```python
from build123d import *

# Parameters (mm, degrees)
F0_W          = 114.3
F0_H          = 21.9340088606
F1_DEPTH      = 76.2
F1_DEPTH_BACK = 76.2
F2_T          = -2.54
F3_R          = 5.08
F4_R          = 6.35
F5_DEPTH      = 12.7
F6_R          = 6.35
F7_DEPTH      = 12.7


with BuildPart() as f1:
    # F0 (on Front) → F1 (new body, two sides)
    with BuildSketch(Plane.XZ) as f1_sk:
        Polygon((-57.15, -101.6), (-76.2, -101.6), (-57.15, -123.5340088606), align=None)
        Polygon((76.2, -101.6), (57.15, -101.6), (57.15, -123.5340088606), align=None)
        Polygon((-76.2, 101.6), (-76.2, -101.6), (-57.15, -101.6), (-57.15, -79.6659911394), (57.15, -79.6659911394), (57.15, -101.6), (76.2, -101.6), (76.2, 101.6), align=None)
        with Locations((0, -90.6329955697)):
            Rectangle(F0_W, F0_H)
        with Locations((0, -112.5670044303)):
            Rectangle(F0_W, F0_H)
    extrude(amount=-F1_DEPTH)
    extrude(f1_sk.sketch, amount=F1_DEPTH_BACK)

    # F2
    f2_openings = [f1.faces().sort_by_distance(p)[0] for p in [
        (0, 0, 101.6),
    ]]
    offset(amount=F2_T, openings=f2_openings)

    # F3
    f3_edges = [f1.edges().sort_by_distance(p)[0] for p in [
        (-66.675, 76.2, -112.567004),
        (-57.15, 0, -123.534009),
        (-66.675, -76.2, -112.567004),
        (-76.2, 0, -101.6),
        (57.15, 0, -123.534009),
        (66.675, 76.2, -112.567004),
        (76.2, 0, -101.6),
        (66.675, -76.2, -112.567004),
    ]]
    fillet(f3_edges, radius=F3_R)

    # F4 (on face) → F5 (join)
    with BuildSketch(Plane(origin=(-76.2, 0, 0), x_dir=(0, -1, 0), z_dir=(-1, 0, 0))):
        with Locations((-44.45, 69.85)):
            Circle(F4_R)
        with Locations((44.45, 69.85)):
            Circle(F4_R)
    extrude(amount=F5_DEPTH)

    # F6 (on face) → F7 (join)
    with BuildSketch(Plane.YZ.offset(76.2)):
        with Locations((-44.45, 69.85)):
            Circle(F6_R)
        with Locations((44.45, 69.85)):
            Circle(F6_R)
    extrude(amount=F7_DEPTH)


solid = f1.part
```
CAD build for the part. Positions are in the model's coordinates, mm. A direction names the side the tool comes from. Coordinates: 2 decimals unless noted, no trailing zeros. Loops run counter-clockwise (first coordinate to the right, second up) from the corner with the lowest first, then second, coordinate; pieces in that order, holes last. Notation, with made-up numbers: (22, 87) - (45, 87) arc R23 ccw to (45, 97) - close; hole circle Ø5 at (80.25, -15.5). An arc over 180 degrees is marked (long way). Use CSV: the item, a comma, the result in double quotes. Start each with the question number.
Q1. 3-axis set-ups, long thin cutter, end or side, ignore diameter. For faces 1 (the cylindrical face through (82.461, -41.036, 75.204)), 2 (the cylindrical face through (-82.461, -47.864, 75.204)), 3 (the cylindrical face through (66.17, 74.75, -110.82)), 4 (the flat face through (74, 34, 101.6)), 5 (the flat face through (-1, 1, -120.994)): which of +Z, -Z, +X, -X, +Y, -Y reach the whole face in a straight line?
Q2. Cut at B-B, the plane y = 32. List the corners of the cut face in (x, z).
Q3. Cut at A-A, the plane z = 58. List the corners of the cut face in (x, y), then the cut area to 3 significant figures.
Q4. Cut at C-C, the plane x = 25. List the corners of the cut face in (y, z).
Q5. Probe probe 1 along X at (y, z) = (4, 25); probe 2 along Z at (x, y) = (3.5, 54). List the from-to ranges inside material, lowest first. Write a range as from..to.
Q6. Two-plate mould, pull along Y, no slides. Class faces 6 (the flat face through (88.9, 44, 70)), 7 (the cylindrical face through (-65.872, 74.672, -111.282)), 8 (the flat face through (-1, -73.66, -8)): +Y half, -Y half, draft (parallel to the pull), parting line (faces both ways), or undercut.
Q7. Drop flat-ended pins along their axis: P1, Ø6, axis at y = 10, z = -13, coming from the -X side; P2, Ø1.5, axis at x = 57, y = 10.5, coming from the +Z side; P3, Ø1.5, axis at y = -21, z = 69.5, coming from the +X side. Give the stop position or say it passes through.
Here are the results:
1,face 1,"+X"
1,face 2,"-X"
1,face 3,"-Z, +X, +Y"
1,face 4,"+Z, +X, -X, +Y, -Y"
1,face 5,"+Z"
2,outline,"(-76.2, -99.7) arc R5.08 ccw to (-74.96, -103.03) - (-58.67, -121.79) arc R5.08 ccw to (-54.83, -123.53) - (54.83, -123.53) arc R5.08 ccw to (58.67, -121.79) - (74.96, -103.03) arc R5.08 ccw to (76.2, -99.7) - (76.2, 101.6) - (73.66, 101.6) - (73.66, -100.65) - (55.99, -120.99) - (-55.99, -120.99) - (-73.66, -100.65) - (-73.66, 101.6) - (-76.2, 101.6) - close"
3,outline,"(-76.2, -76.2) - (76.2, -76.2) - (76.2, 76.2) - (-76.2, 76.2) - close; hole (-73.66, -73.66) - (73.66, -73.66) - (73.66, 73.66) - (-73.66, 73.66) - close"
3,area,"1,520 mm2"
4,outline,"(-76.2, -123.53) - (76.2, -123.53) - (76.2, 101.6) - (73.66, 101.6) - (73.66, -120.99) - (-73.66, -120.99) - (-73.66, 101.6) - (-76.2, 101.6) - close"
5,probe 1,"-76.2..-73.66, 73.66..76.2"
5,probe 2,"-123.53..-120.99"
6,face 6,"draft"
6,face 7,"+Y half"
6,face 8,"undercut"
7,P1,"x = -76.2"
7,P2,"z = -118.97"
7,P3,"x = 76.2"
